Check sheet for the drawn part. Datum: minimum x, y, z corner. Units: mm. A direction names the side the tool comes from. Coordinates: 2 decimals unless noted, no trailing zeros. Write each loop counter-clockwise with the first axis right and the second up, starting at its lowest first coordinate (ties: lowest second). Pieces come first, ordered by that corner, then holes. Notation, with made-up numbers: M -8,14.5 L -1,14.5 A16 ccw -1,18.5 Z; hole C -37.75,21.5 d1. An arc over 180 degrees is marked long. Answer as a JSON object with one key per item and string values. Group by question number.
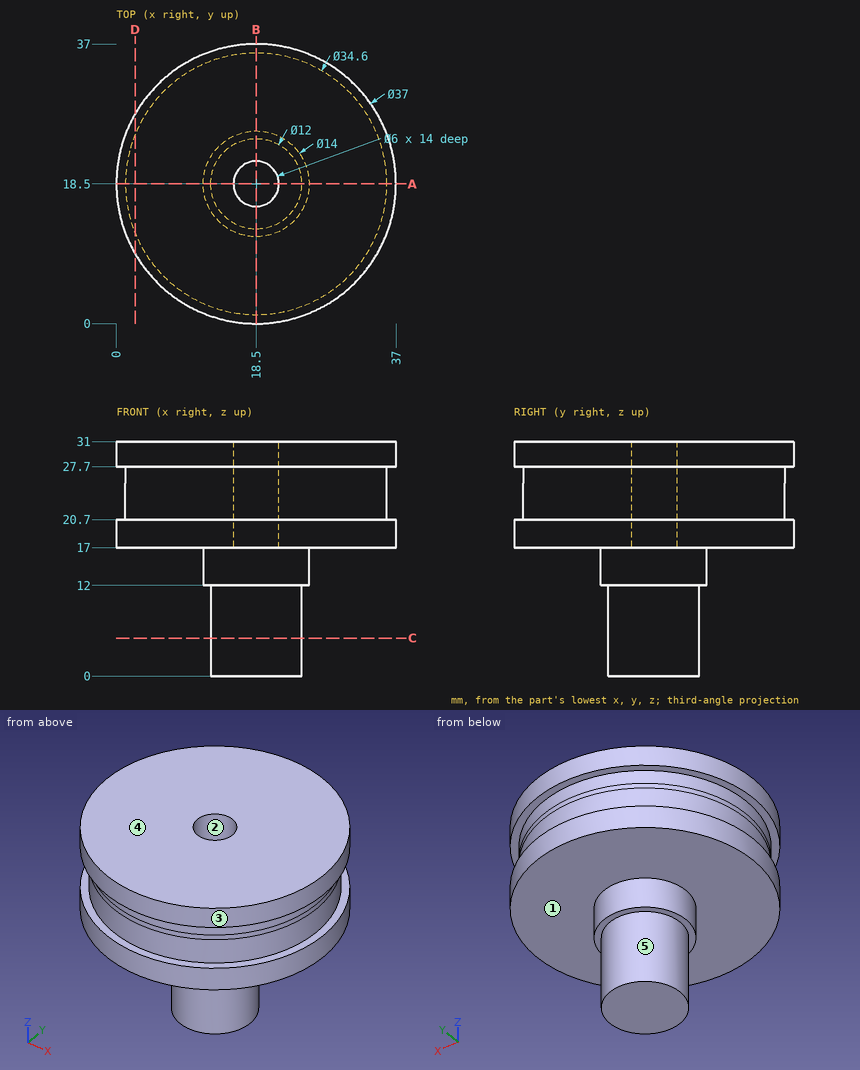
1) Set-up check for the marked faces 4 and 5: record each of +Z, -Z, +X, -X, +Y, -Y from which the full face is reachable in a straight line by a thin tool's end or side.
2) Go/stop test with flat-tipped pins: pin 1 Ø6 at (y, z) = (11.5, 19.5) entering from +X; pin 2 Ø8 at (x, z) = (30.5, 22) entering from -Y; pin 3 Ø15.5 at (x, y) = (17, 16) entering from -Z; pin 4 Ø3 at (x, z) = (28.5, 24) entering from -Y. Record where each tip stops, or that it passes through.
3) Material ranges on probe 1 along Y at (x, z) = (18.5, 21.5); probe 2 along Z at (x, y) = (12, 30.5); probe 3 along Z at (x, y) = (5.5, 7), recorded low to high. Write a range as [from, to].
4) Section check C-C (z = 5). Record the cut outline in (x, y), then the cut area to 3 significant figures.
5) Section check D-D (x = 2.5). Record the cut outline in (y, z).
6) Draft check along X on the marked faces 1, 2 and 3. Enter one of: +X half, -X half, draft (parallel to the pull), parting line (faces both ways), or undercut.
7) Section check A-A (y = 18.5). Record the cut outline in (x, z).
Entries:
{
 "1": {"face 4": "+Z, +X, -X, +Y, -Y", "face 5": "-Z"},
 "2": {"pin 1": "x = 36.56", "pin 2": "y = 1.93", "pin 3": "z = 0", "pin 4": "y = 3.43"},
 "3": {"probe 1": "[1.2, 15.5], [21.5, 35.8]", "probe 2": "[17, 31]", "probe 3": "[17, 20.7], [27.7, 31]"},
 "4": {"outline": "C 18.5,18.5 d12", "area": "113 mm^2"},
 "5": {"outline": "M 9.21,17 L 27.79,17 L 27.79,20.7 L 25.08,20.7 L 25.08,27.7 L 27.79,27.7 L 27.79,31 L 9.21,31 L 9.21,27.7 L 11.92,27.7 L 11.92,20.7 L 9.21,20.7 Z"},
 "6": {"face 1": "draft", "face 2": "undercut", "face 3": "parting line"},
 "7": {"outline": "M 0,17 L 11.5,17 L 11.5,12 L 12.5,12 L 12.5,0 L 24.5,0 L 24.5,12 L 25.5,12 L 25.5,17 L 37,17 L 37,20.7 L 35.8,20.7 L 35.8,27.7 L 37,27.7 L 37,31 L 21.5,31 L 21.5,17 L 15.5,17 L 15.5,31 L 0,31 L 0,27.7 L 1.2,27.7 L 1.2,20.7 L 0,20.7 Z"}
}
